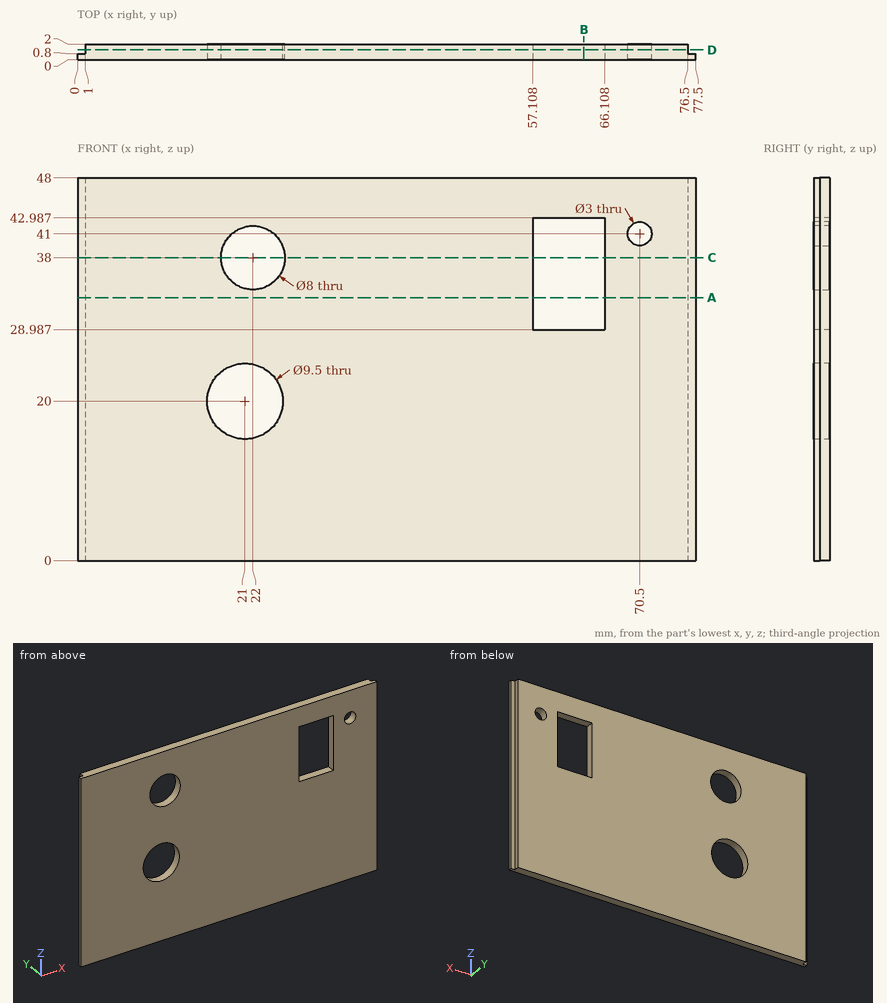
Print and shaded views of the part. All mm, measured from the part's lowest x, y and z. Coordinates: 2 decimals unless noted, no trailing zeros. Loops run counter-clockwise (first coordinate to the right, second up) from the corner with the lowest first, then second, coordinate; pieces in that order, holes last. Notation, with made-up numbers: (52, 47) -> (80, 47) arc R34 cw to (80, 85) -> close; hole circle Ø3 at (41.25, -29). An arc over 180 degrees is marked (long way). Use one line per item in the form item = value. Start each with the question number.
(1) Cut at B-B on x = 63.5. Give the cut face in (y, z).
(2) Cut at C-C on z = 38. Give the cut face in (x, y).
(3) Cut at D-D on y = 1.25. Give the cut face in (x, z), and give its area (3 significant figures).
(4) Probe probe 1 along X at (y, z) = (1.25, 38); probe 2 along X at (y, z) = (1.85, 29.5); probe 3 along X at (y, z) = (0.75, 31.5). List the from-to ranges inside material, lowest first. Write a range as from..to.
(5) Cut at A-A on z = 33. Give the cut face in (x, y).
(6) Flat gauge pins, fed straight in: pin 1 (8.5 mm diameter, centred on x = 21, z = 20, fed in from -Y); pin 2 (0.5 mm diameter, centred on x = 77, z = 26.5, fed in from +Y); pin 3 (1 mm diameter, centred on y = 1.5, z = 20.5, fed in from -X). Where does each tip first touch, or does it go through?
Values:
q1.outline = (0, 0) -> (2, 0) -> (2, 28.99) -> (0, 28.99) -> close; (0, 42.99) -> (2, 42.99) -> (2, 48) -> (0, 48) -> close
q2.outline = (0, 0) -> (18, 0) -> (18, 2) -> (1, 2) -> (1, 0.8) -> (0, 0.8) -> close; (26, 0) -> (57.11, 0) -> (57.11, 2) -> (26, 2) -> close; (66.11, 0) -> (77.5, 0) -> (77.5, 0.8) -> (76.5, 0.8) -> (76.5, 2) -> (66.11, 2) -> close
q3.outline = (1, 0) -> (76.5, 0) -> (76.5, 48) -> (1, 48) -> close; hole circle Ø9.5 at (21, 20); hole circle Ø8 at (22, 38); hole (57.11, 28.99) -> (66.11, 28.99) -> (66.11, 42.99) -> (57.11, 42.99) -> close; hole circle Ø3 at (70.5, 41)
q3.area = 3,370 mm2
q4.probe_1 = 1..18, 26..57.11, 66.11..76.5
q4.probe_2 = 1..57.11, 66.11..76.5
q4.probe_3 = 0..57.11, 66.11..77.5
q5.outline = (0, 0) -> (57.11, 0) -> (57.11, 2) -> (1, 2) -> (1, 0.8) -> (0, 0.8) -> close; (66.11, 0) -> (77.5, 0) -> (77.5, 0.8) -> (76.5, 0.8) -> (76.5, 2) -> (66.11, 2) -> close
q6.pin_1 = through
q6.pin_2 = 0.8
q6.pin_3 = 1
